```python
from build123d import *

# Parameters (mm, degrees)
SKETCH1_R               = 15
SKETCH1_R_2             = 6
BOSS_EXTRUDE1_DEPTH     = 10
CUT_EXTRUDE1_REACH      = 25.452
SKETCH2_W               = 1
SKETCH2_H               = 15
CUT_EXTRUDE2_DEPTH      = 30
CUT_EXTRUDE2_DEPTH_BACK = 30
SKETCH3_R               = 1.6
CUT_EXTRUDE3_START      = -6
SKETCH4_R               = 3.25
CUT_EXTRUDE3_DEPTH      = 30
CUT_EXTRUDE4_START      = -6
CUT_EXTRUDE4_DEPTH      = 30
CUT_EXTRUDE6_REACH      = 25.452
SKETCH10_R              = 2.1
SKETCH11_R              = 2.1
BOSS_EXTRUDE3_DEPTH     = 8


with BuildPart() as part:
    # Sketch1 → Boss-Extrude1 (new body)
    with BuildSketch(Plane.XY):
        Circle(SKETCH1_R)
        Circle(SKETCH1_R_2, mode=Mode.SUBTRACT)
    extrude(amount=BOSS_EXTRUDE1_DEPTH)

    # Sketch2 → Cut-Extrude1 (cut, up to next)
    with BuildSketch(Plane.XY.offset(10), mode=Mode.PRIVATE) as cut_extrude1_sk1:
        with Locations((0, 10.5)):
            Rectangle(SKETCH2_W, SKETCH2_H)
    cut_extrude1_tool1 = extrude(cut_extrude1_sk1.sketch, amount=-CUT_EXTRUDE1_REACH, mode=Mode.PRIVATE) & part.part
    add(cut_extrude1_tool1.solids().sort_by_distance((0, 10.5, 10))[0], mode=Mode.SUBTRACT)

    # Sketch3 → Cut-Extrude2 (cut, two sides: drawn at the far end of the back side and taken through both)
    with BuildSketch(Plane.ZY.offset(-0.5).offset(-CUT_EXTRUDE2_DEPTH_BACK)):
        with Locations(Location((5, 10.991664351, 0), (0, 0, 90))):
            Circle(SKETCH3_R)
    extrude(amount=CUT_EXTRUDE2_DEPTH + CUT_EXTRUDE2_DEPTH_BACK, mode=Mode.SUBTRACT)

    # Sketch4 → Cut-Extrude3 (cut)
    with BuildSketch(Plane.ZY.offset(-0.5).offset(CUT_EXTRUDE3_START)):
        with Locations((5, 10.991664351)):
            Circle(SKETCH4_R)
    extrude(amount=-CUT_EXTRUDE3_DEPTH, mode=Mode.SUBTRACT)

    # Sketch5 → Cut-Extrude4 (cut)
    with BuildSketch(Plane(origin=(-0.5, 0, 0), x_dir=(0, 0, -1), z_dir=(1, 0, 0)).offset(CUT_EXTRUDE4_START)):
        Polygon((-2.2, 9.375083597), (-2.2, 12.608245104), (-5, 14.224825858), (-7.8, 12.608245104), (-7.8, 9.375083597), (-5, 7.758502843), align=None)
    extrude(amount=-CUT_EXTRUDE4_DEPTH, mode=Mode.SUBTRACT)

    # Sketch10 → Cut-Extrude6 (cut, up to next)
    with BuildSketch(Plane.XY.offset(10), mode=Mode.PRIVATE) as cut_extrude6_sk1:
        with Locations((11.31, 0)):
            Circle(SKETCH10_R)
    cut_extrude6_tool1 = extrude(cut_extrude6_sk1.sketch, amount=-CUT_EXTRUDE6_REACH, mode=Mode.PRIVATE) & part.part
    # Sketch10 → Cut-Extrude6 (cut, up to next)
    with BuildSketch(Plane.XY.offset(10), mode=Mode.PRIVATE) as cut_extrude6_sk2:
        with Locations((-11.31, 0)):
            Circle(SKETCH10_R)
    cut_extrude6_tool2 = extrude(cut_extrude6_sk2.sketch, amount=-CUT_EXTRUDE6_REACH, mode=Mode.PRIVATE) & part.part
    add(cut_extrude6_tool1.solids().sort_by_distance((11.31, 0, 10))[0], mode=Mode.SUBTRACT)
    add(cut_extrude6_tool2.solids().sort_by_distance((-11.31, 0, 10))[0], mode=Mode.SUBTRACT)

    # Sketch11 → Boss-Extrude3 (add)
    with BuildSketch(Plane.XY.offset(10)):
        with BuildLine():
            Line((0.5, 14.991664351), (0.5, 5.979130372))
            ThreePointArc((0.5, 5.979130372), (0, -6), (-0.5, 5.979130372))
            Line((-0.5, 5.979130372), (-0.5, 14.991664351))
            ThreePointArc((-0.5, 14.991664351), (0, -15), (0.5, 14.991664351))
        make_face()
        with Locations((11.31, 0)):
            Circle(SKETCH11_R, mode=Mode.SUBTRACT)
        with Locations((-11.31, 0)):
            Circle(SKETCH11_R, mode=Mode.SUBTRACT)
    extrude(amount=BOSS_EXTRUDE3_DEPTH)


solid = part.part
```
Design review of the part built by this model. Coordinates are the model's own, in mm. A direction names the side the tool comes from. Give positions to 0.01 mm unless a question says otherwise; leave off trailing zeros. Loops run counter-clockwise (first coordinate to the right, second up) from the corner with the lowest first, then second, coordinate; pieces in that order, holes last. Notation, with made-up numbers: M 89.5,-9 L 136.5,-9 A17 ccw 136.5,-2 Z; hole C 9.5,-37.5 d7. An arc over 180 degrees is marked long. Return JSON: item names as keys, results as strings. Group by question number.
Item 1: We need section D-D (x = -10). Give the boundary of the cut face in (y, z), and give its area (3 significant figures).
Item 2: Mouldability with a two-part tool opening along Y and no side actions: class faces 6 (the flat face through (-7.121, 12.956, 2.802)), 7 (the flat face through (0.5, 11, 9)), 8 (the cylindrical face through (3.54, 12.52, 4.52)) as released by +Y, released by -Y, zero draft, split by the parting line, or undercut.
Item 3: For probe 1 along X at (y, z) = (0.75, 4.5); probe 2 along X at (y, z) = (10.75, 3); probe 3 along Y at (x, z) = (2, 6.75), list the stretches that pass through material, from the lowest coordinate up.
Item 4: Insertion check: pin 1 Ø10 at (y, z) = (9, 12) entering from +X; pin 2 Ø1.9 at (y, z) = (10.99, 5) entering from -X; pin 3 Ø4 at (y, z) = (10.99, 5) entering from -X; pin 4 Ø8 at (x, z) = (-7.5, 7) entering from -Y. Each pin has a flat end and moves straight along its axis. Give the tip position at first contact, or say it passes through.
Item 5: Tool access review of faces 1 (the flat face through (-0.2, -6.5, 0)), 2 (the flat face through (-0.2, -6.5, 18)), 3 (the flat face through (-0.5, 10, 9)), 4 (the flat face through (-8, 11, 7.8)), 5 (the flat face through (6.5, 9, 5)): name each direction out of +Z, -Z, +X, -X, +Y, -Y from which nothing blocks a thin tool from reaching the whole face with its end or side.
Item 6: We need section A-A (x = -2). Give the boundary of the cut face in (y, z), and give its area (3 significant figures).
Item 7: We need section B-B (y = -3.5). Give the boundary of the cut face in (x, z), and give its area (3 significant figures).
Item 8: We need section C-C (z = 15.5). Give the boundary of the cut face in (x, y), and give its area (3 significant figures).
Output:
{
 "1": {"outline": "M -11.18,0 L -1.64,0 L -1.64,18 L -11.18,18 Z; M 1.64,0 L 11.18,0 L 11.18,2.2 L 9.38,2.2 L 7.76,5 L 9.38,7.8 L 11.18,7.8 L 11.18,18 L 1.64,18 Z", "area": "329 mm^2"},
 "2": {"face 6": "undercut", "face 7": "zero draft", "face 8": "undercut"},
 "3": {"probe 1": "x = -14.98 to -13.27, -9.35 to -5.95, 5.95 to 9.35, 13.27 to 14.98", "probe 2": "x = -6.5 to -0.5, 0.5 to 6.5", "probe 3": "y = -14.87 to -5.66, 5.66 to 14.87"},
 "4": {"pin 1": "stops at x = 14.46", "pin 2": "passes through", "pin 3": "stops at x = -6.5", "pin 4": "stops at y = -14.59"},
 "5": {"face 1": "-Z, +X, -X, +Y, -Y", "face 2": "+Z, +X, -X, +Y, -Y", "face 3": "+Z, -Z, +Y", "face 4": "-X", "face 5": "+X"},
 "6": {"outline": "M -14.87,0 L -5.66,0 L -5.66,18 L -14.87,18 Z; M 5.66,0 L 14.87,0 L 14.87,18 L 5.66,18 Z; hole C 10.99,5 d3.2", "area": "323 mm^2"},
 "7": {"outline": "M -14.59,0 L -4.87,0 L -4.87,18 L -14.59,18 Z; M 4.87,0 L 14.59,0 L 14.59,18 L 4.87,18 Z", "area": "350 mm^2"},
 "8": {"outline": "M -0.5,5.98 L -0.5,14.99 A15 ccw long 0.5,14.99 L 0.5,5.98 A6 cw long Z; hole C -11.31,0 d4.2; hole C 11.31,0 d4.2", "area": "557 mm^2"}
}
